Geometry check sheet. Reference: the model listing, model coordinates, mm. Face numbers are marked on the shaded views. Coordinates: 2 decimals unless noted, no trailing zeros. Loops run counter-clockwise (first coordinate to the right, second up) from the corner with the lowest first, then second, coordinate; pieces in that order, holes last. Notation, with made-up numbers: M 88.25,81.5 L 142.25,81.5 A4 cw 142.25,86.5 Z; hole C 54,-30 d9. An arc over 180 degrees is marked long. Use CSV: the item, a comma, the result in double quotes.
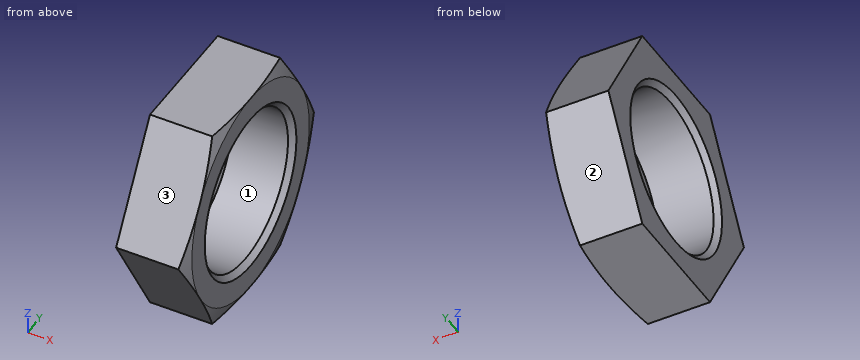
Solid Edge part; units mm, degrees
sketch "Sketch1" plane through (0, 0, 0) normal (0, 0, 1) x (1, 0, 0)
  line L0 (-5, 0) -> (-5, 19.2)
  line L1 (-5, 19.2) -> (4.1426, 19.2)
  line L2 (4.1426, 19.2) -> (5, 16)
  line L3 (5, 16) -> (5, 0)
  line L4 (5, 0) -> (-5, 0)
revolve "RevolvedProtrusion1" add sketch "Sketch1" angle 360 about axis through (5, 0, 0) along (-1, 0, 0)
sketch "Sketch2" plane through (0, 0, 0) normal (0, 0, 1) x (1, 0, 0)
  line L0 (-5, 0) -> (-5, 12.5)
  line L1 (-5, 12.5) -> (-4.188, 11.688)
  line L2 (-4.188, 11.688) -> (4.188, 11.688)
  line L3 (4.188, 11.688) -> (5, 12.5)
  line L4 (5, 12.5) -> (5, 0)
  line L5 (5, 0) -> (-5, 0)
revolve "RevolvedCutout1" cut sketch "Sketch2" angle 360 about axis through (5, 0, 0) along (-1, 0, 0)
cosmetic_thread "Thread1"
sketch "Sketch3" plane through (0, 0, 0) normal (1, 0, 0) x (0, 1, 0)
  line L0 (-32, 32) -> (-32, -32)
  line L1 (-32, -32) -> (32, -32)
  line L2 (32, -32) -> (32, 32)
  line L3 (32, 32) -> (-32, 32)
  line L4 (9.2376, 16) -> (-9.2376, 16)
  line L5 (-9.2376, 16) -> (-18.4752, 0)
  line L6 (-18.4752, 0) -> (-9.2376, -16)
  line L7 (-9.2376, -16) -> (9.2376, -16)
  line L8 (9.2376, -16) -> (18.4752, 0)
  line L9 (18.4752, 0) -> (9.2376, 16)
extrude "ExtrudedCutout_1" cut sketch "Sketch3" against normal blind 10 and the other way blind 10
1. Gauge pin test, flat ends, axial feed: P1, Ø14, axis at y = 0, z = 0, coming from the +X side; P2, Ø3, axis at y = -9.5, z = -4.5, coming from the -X side; P3, Ø3, axis at x = -2, z = -10, coming from the +Y side; P4, Ø1, axis at x = 2.5, z = -2, coming from the -Y side. Record the tip position at first contact, or that the pin passes through.
The answers:
P1,"through"
P2,"x = -4.51"
P3,"y = 13.57"
P4,"y = -17.61"
2. Release check for a two-part mould opening along Y. For the marked faces 1, 2 and 3 record: +Y half, -Y half, draft (parallel to the pull), parting line (faces both ways), or undercut.
The answers:
face 1,"undercut"
face 2,"+Y half"
face 3,"-Y half"
3. Thickness scan on line 1 (Z direction, x = 1.5, y = 0); line 2 (Y direction, x = 0.5, z = 0); line 3 (Y direction, x = 3.25, z = 9.5). Record the ranges inside material, lowest first. Write a range as [from, to].
The answers:
line 1,"[-16, -11.69], [11.69, 16]"
line 2,"[-18.48, -11.69], [11.69, 18.48]"
line 3,"[-12.99, -6.81], [6.81, 12.99]"
4. Section check A-A, the plane x = -1.25. Record the cut outline in (y, z).
The answers:
outline,"M -18.48,0 L -9.24,-16 L 9.24,-16 L 18.48,0 L 9.24,16 L -9.24,16 Z; hole C 0,0 d23.38"
